Autodesk Inventor part; units mm, degrees
ref_plane "YZ Plane" through (0, 0, 0) normal (1, 0, 0) x (0, 1, 0)
ref_plane "XZ Plane" through (0, 0, 0) normal (0, 1, 0) x (-1, 0, 0)
ref_plane "XY Plane" through (0, 0, 0) normal (0, 0, 1) x (1, 0, 0)
sketch "Sketch1" plane through (0, 0, 0) normal (0, 0, 1) x (1, 0, 0)
  arc A0 (-5.5597, 8.9556) -> (-9.9691, -3.4248) centre (0, 0) ccw
  line L0 (0, 0) -> (0, 33.782)
  line L1 (0, 33.782) -> (-5.5597, 33.782)
  line L2 (-5.5597, 33.782) -> (-5.5597, 8.9556)
  line L3 (0, 0) -> (0, -2.735)
  arc A1 (0, 9.017) -> (-8.3413, -3.4248) centre (0, 0) ccw
  line L4 (-9.9691, -3.4248) -> (-8.3413, -3.4248)
  dimension "d1" = 21.082
  dimension "d2" = 1.524
  dimension "d12" = 33.782
revolve "Revolution1" add sketch "Sketch1" angle 360 about axis through (0, 0, 0) along (0, 1, 0)
sketch "Sketch4" plane through (0, 33.782, 0) normal (0, 1, 0) x (1, 0, 0)
  circle A0 centre (0, 0) radius 2.8575
  dimension "d4" = 5.715
extrude "Extrusion1" cut sketch "Sketch4" against normal blind 1.27
sketch "Sketch5" plane through (0, 0, 0) normal (1, 0, 0) x (0, 1, 0)
  line L0 (-3.4248, -9.9691) -> (-3.4248, 9.9691)
  circle A0 centre (-3.4248, 0) radius 4.064
  point P0 (0, 0)
  dimension "d7" = 8.128
extrude "Extrusion2" cut sketch "Sketch5" along normal mid plane 2540
sketch "Sketch7" plane through (0, 0, 0) normal (0, 0, 1) x (1, 0, 0)
  line L0 (7.2843, -3.4248) -> (-7.2843, -3.4248)
  circle A0 centre (0, -3.4248) radius 4.1452
  point P0 (0, 0)
extrude "Extrusion3" cut sketch "Sketch7" along normal mid plane 2540
properties part number "caster sumo jeffrey p"
Verification items for the finished model (mm, model axes). A direction names the side the tool comes from. Coordinates: 2 decimals unless noted, no trailing zeros. Loops run counter-clockwise (first coordinate to the right, second up) from the corner with the lowest first, then second, coordinate; pieces in that order, holes last. Notation, with made-up numbers: (20, 52.5) -> (58, 52.5) arc R10 ccw to (58, 69.5) -> close; hole circle Ø2 at (88, 2). An arc over 180 degrees is marked (long way). Answer in a Markdown table with one row per item.
1) Access from +Z, -Z, +X, -X, +Y, -Y to the whole of each face (thin tool, end or side, straight path). Record for faces 1 (the face through (6.7, -3.425, -6.5)), 2 (the face through (0, 32.512, 0)).
The answers:
| item | result |
|---|---|
| face 1 | +Z, -Z, +X, -X, -Y |
| face 2 | +Y |
2) Section check A-A (y = 12.5). Record the cut outline in (x, z).
The answers:
| item | result |
|---|---|
| outline | circle Ø11.12 at (0, 0) |
3) Draft check along Z on faces 3 (the face through (-5.136, 21.195, 2.129)), 4 (the face through (2.726, 33.156, -0.858)), 5 (the face through (-6.6, -3.425, -6.5)). Enter one of: released by +Z, released by -Z, zero draft, split by the parting line, or undercut.
The answers:
| item | result |
|---|---|
| face 3 | split by the parting line |
| face 4 | undercut |
| face 5 | zero draft |
4) Depth check by flat-ended pin: P1, Ø5, axis at y = 30, z = 0, coming from the -X side; P2, Ø3, axis at x = -2.5, y = 9.5, coming from the -Z side; P3, Ø5, axis at x = 5.5, z = -1, coming from the +Y side; P4, Ø5, axis at x = 0, z = 0, coming from the +Y side. Enter the tip coordinate at first touch or a pass-through.
The answers:
| item | result |
|---|---|
| P1 | stops at x = -5.56 |
| P2 | stops at z = -6.47 |
| P3 | stops at y = 33.78 |
| P4 | stops at y = 32.51 |
5) Scan lines: line 1 along Z through (x, y) = (0, 33.25); line 2 along Z through (x, y) = (-2, 23); line 3 along Y through (x, z) = (7.5, -2.25). Record each from-to range of solid material in increasing order. Write a range as from..to.
The answers:
| item | result |
|---|---|
| line 1 | z = -5.56..-2.86, 2.86..5.56 |
| line 2 | z = -5.19..5.19 |
| line 3 | y = 4.47..7.06 |
